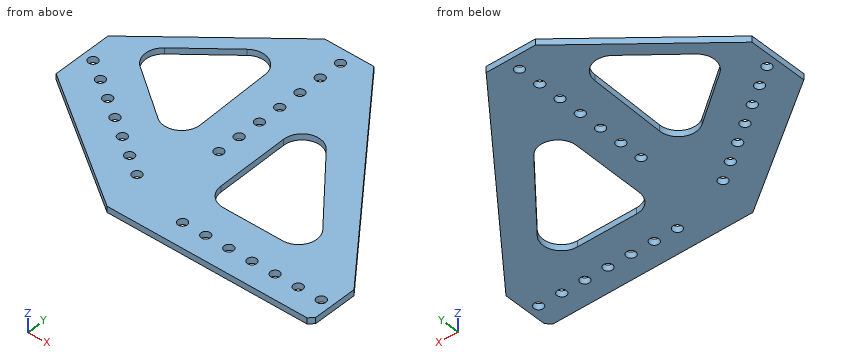
from build123d import *

# Parameters (mm, degrees)
SKETCH1_W           = 25.4
SKETCH1_H           = 90.039220871
SKETCH1_R           = 2.54
SKETCH1_W_2         = 88.349378458
SKETCH1_H_2         = 25.4
BOSS_EXTRUDE3_DEPTH = 3.302
CHAMFER5_SIZE       = 114.3
CHAMFER5_SIZE2      = 89.30094711
CHAMFER6_SIZE       = 50.8
CHAMFER6_SIZE2      = 72.549918742
CHAMFER7_SIZE       = 68.58
CHAMFER7_SIZE2      = 57.545452706
CHAMFER10_SIZE      = 2.54
CUT_EXTRUDE1_DEPTH  = 3.302
FILLET1_R           = 10
FILLET2_R           = 10
FILLET3_R           = 10
FILLET4_R           = 10
FILLET5_R           = 10
FILLET6_R           = 10


with BuildPart() as part:
    # Sketch1 → Boss-Extrude3 (new body)
    with BuildSketch(Plane.XY):
        Polygon((-30.387651704, 9.581189779), (-96.521251531, 55.888434907), (-96.521251531, 0), (0, 0), (0, 25.4), (88.349378458, 25.4), (88.349378458, 140.839220871), (0, 140.839220871), (0, 50.8), (-25.4, 50.8), (-25.4, 140.839220871), (-96.521251531, 140.839220871), (-96.521251531, 86.896109461), (-15.818810221, 30.387651704), align=None)
        with Locations((-12.7, 95.819610436)):
            Rectangle(SKETCH1_W, SKETCH1_H)
        with Locations((-12.7, 57.15)):
            Circle(SKETCH1_R, mode=Mode.SUBTRACT)
        with Locations((-12.7, 69.85)):
            Circle(SKETCH1_R, mode=Mode.SUBTRACT)
        with Locations((-12.7, 82.55)):
            Circle(SKETCH1_R, mode=Mode.SUBTRACT)
        with Locations((-12.7, 95.25)):
            Circle(SKETCH1_R, mode=Mode.SUBTRACT)
        with Locations((-12.7, 107.95)):
            Circle(SKETCH1_R, mode=Mode.SUBTRACT)
        with Locations((-12.7, 120.65)):
            Circle(SKETCH1_R, mode=Mode.SUBTRACT)
        with Locations((-12.7, 133.35)):
            Circle(SKETCH1_R, mode=Mode.SUBTRACT)
        Polygon((-96.521251531, 86.896109461), (-96.521251531, 55.888434907), (-30.387651704, 9.581189779), (-15.818810221, 30.387651704), align=None)
        with Locations((-38.708077406, 30.911051854)):
            Circle(SKETCH1_R, mode=Mode.SUBTRACT)
        with Locations((-28.304846444, 23.626631112)):
            Circle(SKETCH1_R, mode=Mode.SUBTRACT)
        with Locations((-49.111308369, 38.195472596)):
            Circle(SKETCH1_R, mode=Mode.SUBTRACT)
        with Locations((-59.514539331, 45.479893337)):
            Circle(SKETCH1_R, mode=Mode.SUBTRACT)
        with Locations((-69.917770294, 52.764314079)):
            Circle(SKETCH1_R, mode=Mode.SUBTRACT)
        with Locations((-80.321001256, 60.048734821)):
            Circle(SKETCH1_R, mode=Mode.SUBTRACT)
        with Locations((-90.724232219, 67.333155562)):
            Circle(SKETCH1_R, mode=Mode.SUBTRACT)
        with Locations((44.174689229, 12.7)):
            Rectangle(SKETCH1_W_2, SKETCH1_H_2)
        with Locations((6.35, 12.7)):
            Circle(SKETCH1_R, mode=Mode.SUBTRACT)
        with Locations((19.05, 12.7)):
            Circle(SKETCH1_R, mode=Mode.SUBTRACT)
        with Locations((31.75, 12.7)):
            Circle(SKETCH1_R, mode=Mode.SUBTRACT)
        with Locations((44.45, 12.7)):
            Circle(SKETCH1_R, mode=Mode.SUBTRACT)
        with Locations((57.15, 12.7)):
            Circle(SKETCH1_R, mode=Mode.SUBTRACT)
        with Locations((69.85, 12.7)):
            Circle(SKETCH1_R, mode=Mode.SUBTRACT)
        with Locations((82.55, 12.7)):
            Circle(SKETCH1_R, mode=Mode.SUBTRACT)
    extrude(amount=BOSS_EXTRUDE3_DEPTH)

    # Chamfer5
    chamfer5_edges = [part.edges().sort_by_distance(p)[0] for p in [
        (88.349378458, 140.839220871, 1.651),
    ]]
    chamfer5_side = [part.faces().sort_by_distance(p)[0] for p in [
        (88.349378458, 70.419610435, 1.651),
    ]]
    chamfer(chamfer5_edges, length=CHAMFER5_SIZE, length2=CHAMFER5_SIZE2, reference=chamfer5_side[0])

    # Chamfer6
    chamfer6_edges = [part.edges().sort_by_distance(p)[0] for p in [
        (-96.521251531, 0, 1.651),
    ]]
    chamfer6_side = [part.faces().sort_by_distance(p)[0] for p in [
        (-96.521251531, 70.419610435, 1.651),
    ]]
    chamfer(chamfer6_edges, length=CHAMFER6_SIZE, length2=CHAMFER6_SIZE2, reference=chamfer6_side[0])

    # Chamfer7
    chamfer7_edges = [part.edges().sort_by_distance(p)[0] for p in [
        (-96.521251531, 140.839220871, 1.651),
    ]]
    chamfer7_side = [part.faces().sort_by_distance(p)[0] for p in [
        (-48.736410091, 140.839220871, 1.651),
    ]]
    chamfer(chamfer7_edges, length=CHAMFER7_SIZE, length2=CHAMFER7_SIZE2, reference=chamfer7_side[0])

    # Chamfer10
    chamfer10_edges = [part.edges().sort_by_distance(p)[0] for p in [
        (88.349378458, 0, 1.651),
    ]]
    chamfer(chamfer10_edges, length=CHAMFER10_SIZE)

    # Sketch2 → Cut-Extrude1 (cut)
    with BuildSketch(Plane.XY.offset(3.302)):
        Polygon((-31.967710472, 127.732145748), (-83.765850495, 84.732254389), (-29.117573581, 44.458580926), align=None)
        Polygon((1.745305047, 109.142640029), (2.853527199, 30.951410442), (66.547890767, 30.951410442), align=None)
    extrude(amount=-CUT_EXTRUDE1_DEPTH, mode=Mode.SUBTRACT)

    # Fillet1
    fillet1_edges = [part.edges().sort_by_distance(p)[0] for p in [
        (2.853527199, 30.951410442, 1.651),
    ]]
    fillet(fillet1_edges, radius=FILLET1_R)

    # Fillet2
    fillet2_edges = [part.edges().sort_by_distance(p)[0] for p in [
        (-29.117573581, 44.458580926, 1.651),
    ]]
    fillet(fillet2_edges, radius=FILLET2_R)

    # Fillet3
    fillet3_edges = [part.edges().sort_by_distance(p)[0] for p in [
        (66.547890767, 30.951410442, 1.651),
    ]]
    fillet(fillet3_edges, radius=FILLET3_R)

    # Fillet4
    fillet4_edges = [part.edges().sort_by_distance(p)[0] for p in [
        (1.745305047, 109.142640029, 1.651),
    ]]
    fillet(fillet4_edges, radius=FILLET4_R)

    # Fillet5
    fillet5_edges = [part.edges().sort_by_distance(p)[0] for p in [
        (-31.967710472, 127.732145748, 1.651),
    ]]
    fillet(fillet5_edges, radius=FILLET5_R)

    # Fillet6
    fillet6_edges = [part.edges().sort_by_distance(p)[0] for p in [
        (-83.765850495, 84.732254389, 1.651),
    ]]
    fillet(fillet6_edges, radius=FILLET6_R)


solid = part.part
Build history of the part. All positions in model axes, mm. Round coordinates to 2 decimals unless told otherwise and drop trailing zeros. Write each loop counter-clockwise with the first axis right and the second up, starting at its lowest first coordinate (ties: lowest second). Pieces come first, ordered by that corner, then holes. Notation, with made-up numbers: (23.25, 0) -> (36.25, 0) arc R15 cw to (36.25, 5) -> close; hole circle Ø5 at (-27, 45). An arc over 180 degrees is marked (long way). Write item = value, one per line.
(1) Band-saw the part on C-C (y = 100). Give the cut face in (x, z).
Answer:
outline = (-76.61, 0) -> (-65.37, 0) -> (-65.37, 3.3) -> (-76.61, 3.3) -> close; (-31.02, 0) -> (30.96, 0) -> (30.96, 3.3) -> (-31.02, 3.3) -> close
(2) Band-saw the part on A-A (x = -12.7). State how many separate pieces and enclosed holes the cut face has, then the cut area to 3 significant figures.
Answer:
separate_pieces = 8
enclosed_holes = 0
area = 348 mm2
(3) Band-saw the part on D-D (x = 23.5). Give the cut face in (y, z), then the cut area to 3 significant figures.
Answer:
outline = (0, 0) -> (30.95, 0) -> (30.95, 3.3) -> (0, 3.3) -> close; (82.89, 0) -> (109.54, 0) -> (109.54, 3.3) -> (82.89, 3.3) -> close
area = 190 mm2
(4) Probe L1, parallel to X at y = 67, z = 2.9; L2, parallel to X at y = 80.5, z = 1.55; L3, parallel to X at y = 110, z = 0.55. List the from-to ranges inside material, lowest first.
Answer:
L1 = -96.52 to -93.24, -88.21 to -59.7, -29.89 to 2.34, 36.67 to 56.74
L2 = -96.52 to -76.37, -30.35 to -14.2, -11.2 to 2.15, 25.48 to 46.19
L3 = -64.69 to -53.33, -31.72 to -14.2, -11.2 to 23.14
(5) Flat gauge pin, fed straight in: pin 1 (4.5 mm diameter, centred on x = -59.51, y = 45.48, fed in from +Z). Where does the tip first touch, or does it go through?
Answer:
pin_1 = through
